```python
from build123d import *

# Parameters (mm, degrees)
SKETCH1_R           = 9
BOSS_EXTRUDE1_DEPTH = 30
SKETCH2_W           = 10
SKETCH2_H           = 10
CUT_EXTRUDE1_DEPTH  = 33.588341474
CUT_EXTRUDE3_DEPTH  = 33.588341474
CUT_EXTRUDE4_START  = -8
SKETCH4_R           = 1.5
CUT_EXTRUDE4_DEPTH  = 41.588341621
SKETCH6_R           = 0.625
CUT_EXTRUDE5_DEPTH  = 10
CUT_EXTRUDE6_REACH  = 25.707
SKETCH7_W           = 3
SKETCH7_H           = 2
SKETCH8_R           = 0.9
CUT_EXTRUDE7_DEPTH  = 5


with BuildPart() as part:
    # Sketch1 → Boss-Extrude1 (new body)
    with BuildSketch(Plane.XY):
        Circle(SKETCH1_R)
    extrude(amount=-BOSS_EXTRUDE1_DEPTH)

    # Sketch2 → Cut-Extrude1 (cut, symmetric)
    with BuildSketch(Plane(origin=(0, 0, 0), x_dir=(1, 0, 0), z_dir=(0, 1, 0))):
        with Locations((0, 25)):
            Rectangle(SKETCH2_W, SKETCH2_H)
    cut_extrude1 = extrude(amount=CUT_EXTRUDE1_DEPTH, both=True, mode=Mode.SUBTRACT)

    # Sketch5 → Cut-Extrude3 (cut, symmetric)
    with BuildSketch(Plane(origin=(0, 0, 0), x_dir=(0, 0, -1), z_dir=(1, 0, 0))):
        with BuildLine():
            Line((20, 7.483314774), (30, 7.483314774))
            Line((30, 7.483314774), (30, 0))
            ThreePointArc((30, 0), (26.031389946, 5.119910176), (20, 7.483314774))
        make_face()
    cut_extrude3 = extrude(amount=CUT_EXTRUDE3_DEPTH, both=True, mode=Mode.SUBTRACT)

    # Sketch4 → Cut-Extrude4 (cut)
    with BuildSketch(Plane(origin=(0, 0, 0), x_dir=(0, 0, -1), z_dir=(1, 0, 0)).offset(CUT_EXTRUDE4_START)):
        with Locations((26, 0)):
            Circle(SKETCH4_R)
    cut_extrude4 = extrude(amount=CUT_EXTRUDE4_DEPTH, mode=Mode.SUBTRACT)

    # Mirror1: Cut-Extrude1, Cut-Extrude3, Cut-Extrude4 across plane
    add(cut_extrude1.mirror(Plane.XY.offset(-15)), mode=Mode.SUBTRACT)
    add(cut_extrude3.mirror(Plane.XY.offset(-15)), mode=Mode.SUBTRACT)
    add(cut_extrude4.mirror(Plane.XY.offset(-15)), mode=Mode.SUBTRACT)

    # Sketch6 → Cut-Extrude5 (cut)
    with BuildSketch(Plane.XY.offset(-10)):
        with Locations((0, 7.5)):
            Circle(SKETCH6_R)
    extrude(amount=-CUT_EXTRUDE5_DEPTH, mode=Mode.SUBTRACT)

    # Sketch7 → Cut-Extrude6 (cut, up to next)
    with BuildSketch(Plane.XY.offset(-10), mode=Mode.PRIVATE) as cut_extrude6_sk1:
        with Locations((0, -9)):
            Rectangle(SKETCH7_W, SKETCH7_H)
    cut_extrude6_tool1 = extrude(cut_extrude6_sk1.sketch, amount=-CUT_EXTRUDE6_REACH, mode=Mode.PRIVATE) & part.part
    add(cut_extrude6_tool1.solids().sort_by_distance((0, -9, -10))[0], mode=Mode.SUBTRACT)

    # Sketch8 → Cut-Extrude7 (cut)
    with BuildSketch(Plane.XZ.offset(8)):
        with Locations(Location((0, -15, 0), (0, 0, 270))):
            Circle(SKETCH8_R)
    extrude(amount=-CUT_EXTRUDE7_DEPTH, mode=Mode.SUBTRACT)


solid = part.part
```
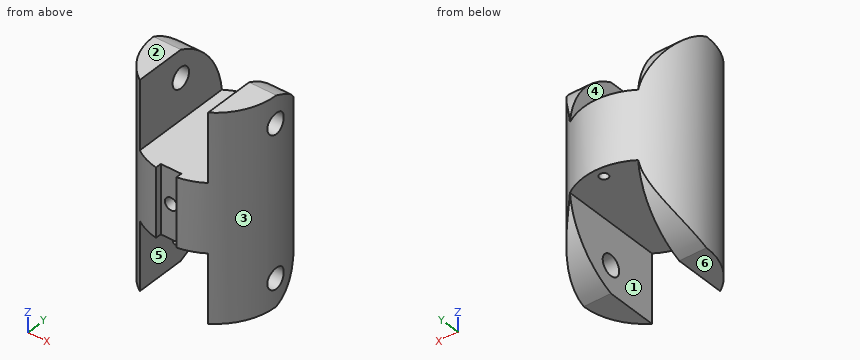
CAD build for the part. Positions are in the model's coordinates, mm. Face numbers are marked on the shaded views. A direction names the side the tool comes from. Coordinates: 2 decimals unless noted, no trailing zeros. Write each loop counter-clockwise with the first axis right and the second up, starting at its lowest first coordinate (ties: lowest second). Pieces come first, ordered by that corner, then holes. Notation, with made-up numbers: (32.5, 66) -> (74.5, 66) arc R21 cw to (74.5, 98) -> close; hole circle Ø11 at (20, 15). An arc over 180 degrees is marked (long way). Return JSON: item names as keys, results as strings. Group by question number.
Q1. Pull direction X, two halves, no side cores. Call the marked faces 1, 2 and 3: released by +X, released by -X, zero draft, split by the parting line, or undercut.
Q2. Cut at D-D, the plane y = 3.25. Give the cut face in (x, z), then the cut area to 3 significant figures.
Q3. Cut at A-A, the plane z = -15. Give the cut face in (x, y) (3 decimals).
Q4. Flat gauge pins, fed straight in: pin 1 (4 mm diameter, centred on y = 0, z = -4, fed in from +X); pin 2 (8 mm diameter, centred on x = 0, y = -1, fed in from +Z); pin 3 (2 mm diameter, centred on y = -3.5, z = -4.5, fed in from -X); pin 4 (0.9 mm diameter, centred on x = 0, z = -15, fed in from -Y). Where does each tip first touch, or does it go through?
Q5. Which spindle directions (+Z, -Z, +X, -X, +Y, -Y) get a long thin tool onto all of the face, cutting with end or side? Do the marked faces 4, 5 and 6. Say none if no direction does.
Q6. Cut at C-C, the plane z = -3.5. Give the cut face in (x, y).
Q7. Cut at B-B, the plane x = 0. Give the cut face in (y, z) (3 decimals).
Q8. Drill centre lines: line 1 (Z direction, x = 6.85, y = 0); line 2 (X direction, y = 0, z = -20.5); line 3 (X direction, y = -5, z = -5). Where is each one in solid material? Low to high.
Returned:
{
 "1": {"face 1": "undercut", "face 2": "zero draft", "face 3": "split by the parting line"},
 "2": {"outline": "(-8.39, -28.02) -> (-5, -28.02) -> (-5, -20) -> (5, -20) -> (5, -28.02) -> (8.39, -28.02) -> (8.39, -1.98) -> (5, -1.98) -> (5, -10) -> (-5, -10) -> (-5, -1.98) -> (-8.39, -1.98) -> close", "area": "277 mm2"},
 "3": {"outline": "(-1.5, -8.874) -> (-1.5, -8) -> (-0.9, -8) -> (-0.9, -3) -> (0.9, -3) -> (0.9, -8) -> (1.5, -8) -> (1.5, -8.874) arc R9 ccw (long way) to start; hole circle Ø1.25 at (0, 7.5)"},
 "4": {"pin 1": "stops at x = 9", "pin 2": "stops at z = -10", "pin 3": "stops at x = -8.65", "pin 4": "stops at y = -3"},
 "5": {"face 4": "+Z, +Y, -Y", "face 5": "-Z, +Y, -Y", "face 6": "-Z, +X, -X, +Y, -Y"},
 "6": {"outline": "(-8, -1.41) -> (-8, 1.41) -> (-5, 1.41) -> (-5, 4.75) -> (-7.64, 4.75) arc R9 ccw to (-5, -7.48) -> (-5, -1.41) -> close; (5, -7.48) arc R9 ccw to (8.89, -1.41) -> (5, -1.41) -> close; (5, 1.41) -> (8.89, 1.41) arc R9 ccw to (7.64, 4.75) -> (5, 4.75) -> close"},
 "7": {"outline": "(-8, -20) -> (6.875, -20) -> (6.875, -10) -> (-8, -10) -> (-8, -14.1) -> (-3, -14.1) -> (-3, -15.9) -> (-8, -15.9) -> close; (8.125, -20) -> (9, -20) -> (9, -10) -> (8.125, -10) -> close"},
 "8": {"line 1": "z = -30 to -27.5, -24.5 to -5.5, -2.5 to 0", "line 2": "x = -9 to -5, 5 to 9", "line 3": "x = -7.48 to -5, 5 to 7.48"}
}
